```python
from build123d import *

# Parameters (mm, degrees)
SKETCH1_R           = 5
SKETCH1_R_2         = 3
BOSS_EXTRUDE1_DEPTH = 5
CHAMFER1_SIZE       = 1.5
SKETCH2_R           = 11
SKETCH2_R_2         = 5
SKETCH2_R_3         = 1.5
BOSS_EXTRUDE2_DEPTH = 1


with BuildPart() as part:
    # Sketch1 → Boss-Extrude1 (new body)
    with BuildSketch(Plane(origin=(0, 0, 0), x_dir=(1, 0, 0), z_dir=(0, 1, 0))):
        Circle(SKETCH1_R)
        Circle(SKETCH1_R_2, mode=Mode.SUBTRACT)
    extrude(amount=BOSS_EXTRUDE1_DEPTH)

    # Chamfer1
    chamfer1_edges = [part.edges().sort_by_distance(p)[0] for p in [
        (-5, 5, 0),
    ]]
    chamfer(chamfer1_edges, length=CHAMFER1_SIZE)

    # Sketch2 → Boss-Extrude2 (add)
    with BuildSketch(Plane.XZ):
        Circle(SKETCH2_R)
        Circle(SKETCH2_R_2, mode=Mode.SUBTRACT)
        with Locations((0, 8)):
            Circle(SKETCH2_R_3, mode=Mode.SUBTRACT)
        with Locations((-8, 0)):
            Circle(SKETCH2_R_3, mode=Mode.SUBTRACT)
        with Locations((0, -8)):
            Circle(SKETCH2_R_3, mode=Mode.SUBTRACT)
        with Locations((8, 0)):
            Circle(SKETCH2_R_3, mode=Mode.SUBTRACT)
    extrude(amount=-BOSS_EXTRUDE2_DEPTH)


solid = part.part
```
Build history of the part. All positions in model axes, mm. A direction names the side the tool comes from. Give positions to 0.01 mm unless a question says otherwise; leave off trailing zeros. Order: outer loops, then holes, each group sorted by start corner. A loop starts at its lowest first (then second) coordinate and runs counter-clockwise, first axis right, second up. Notation, with made-up numbers: M -38.5,-10 L 19.5,-10 A23 cw 19.5,12 Z; hole C -8,-8.5 d10. An arc over 180 degrees is marked long. Write item = value, one per line. Start each with the question number.
(1) Which spindle directions (+Z, -Z, +X, -X, +Y, -Y) get a long thin tool onto all of the face, cutting with end or side? Do faces 1 (the flat face through (5, 1, -2)), 2 (the cylindrical face through (-9.5, 0.49, 0.07)). Say none if no direction does.
(2) Probe L1, parallel to Z at x = 0, y = 0.4; L2, parallel to Z at x = 0, y = 1.2. List the from-to ranges inside material, lowest first. Write a range as [from, to].
(3) Two-plate mould, pull along X, no slides. Class faces 3 (the flat face through (2.3, 0, -2.3)), 4 (the cylindrical face through (6.5, 0.49, 0.07)), 5 (the cylindrical face through (-1.08, 2.23, 4.88)): released by +X, released by -X, zero draft, split by the parting line, or undercut.
(4) Slice it at C-C on z = -7. Write the cut outline in (x, y).
(5) Pin check, flat tips, straight feed: pin 1 Ø3 at (x, y) = (3, 1) entering from +Z; pin 2 Ø2 at (y, z) = (4, 0) entering from -X. Stop position of each tip, or through.
(6) Slice it at D-D on x = 8. Write the cut outline in (y, z), plus the area to 3 significant figures.
(7) Slice it at B-B on x = 0. Write the cut outline in (y, z).
(8) Slice it at A-A on z = 0. Write the cut outline in (x, y).
Responses:
q1.face_1 = +Y
q1.face_2 = +Y, -Y
q2.L1 = [-11, -9.5], [-6.5, -3], [3, 6.5], [9.5, 11]
q2.L2 = [-5, -3], [3, 5]
q3.face_3 = zero draft
q3.face_4 = undercut
q3.face_5 = split by the parting line
q4.outline = M -8.49,0 L -1.12,0 L -1.12,1 L -8.49,1 Z; M 1.12,0 L 8.49,0 L 8.49,1 L 1.12,1 Z
q5.pin_1 = 10.9
q5.pin_2 = -5
q6.outline = M 0,-7.55 L 1,-7.55 L 1,-1.5 L 0,-1.5 Z; M 0,1.5 L 1,1.5 L 1,7.55 L 0,7.55 Z
q6.area = 12.1 mm2
q7.outline = M 0,-11 L 1,-11 L 1,-9.5 L 0,-9.5 Z; M 0,-6.5 L 1,-6.5 L 1,-5 L 3.5,-5 L 5,-3.5 L 5,-3 L 0,-3 Z; M 0,3 L 5,3 L 5,3.5 L 3.5,5 L 1,5 L 1,6.5 L 0,6.5 Z; M 0,9.5 L 1,9.5 L 1,11 L 0,11 Z
q8.outline = M -11,0 L -9.5,0 L -9.5,1 L -11,1 Z; M -6.5,0 L -3,0 L -3,5 L -3.5,5 L -5,3.5 L -5,1 L -6.5,1 Z; M 3,0 L 6.5,0 L 6.5,1 L 5,1 L 5,3.5 L 3.5,5 L 3,5 Z; M 9.5,0 L 11,0 L 11,1 L 9.5,1 Z
